Verification items for the finished model (mm, model axes). A direction names the side the tool comes from. Give positions to 0.01 mm unless a question says otherwise; leave off trailing zeros. Order: outer loops, then holes, each group sorted by start corner. A loop starts at its lowest first (then second) coordinate and runs counter-clockwise, first axis right, second up.
(1) Mould release check, pull along Y, two halves, no side actions. Record for faces 3 (the face through (-18, 24, 0)), 4 (the face through (-0.78, -22.43, -12.4)), 5 (the face through (-1, -25, -7)): pulls with the +Y half, pulls with the -Y half, needs draft (parallel to the pull), parting line crosses it, or undercut.
(2) Sectioned sample at B-B on y = -18. Record the cut outline in (x, z).
(3) Sectioned sample at A-A on z = -5. Record the cut outline in (x, y).
(4) Access from +Z, -Z, +X, -X, +Y, -Y to the whole of each face (thin tool, end or side, straight path). Record for faces 1 (the face through (-57.43, 22.4, -5.58)), 2 (the face through (60, 0, -7)).
(5) Sectioned sample at C-C on x = 18. Record the cut outline in (y, z).
(6) Scan lines: L1, parallel to X at y = -8, z = -3; L2, parallel to Y at x = -41.5, z = -7.75; L3, parallel to Z at x = 53, y = 2.5. Record each from-to range of solid material in increasing order.
(7) Gauge pin test, flat end, axial feed: pin 1 (1.5 mm diameter, centred on x = 18, y = -5.5, fed in from +Z). Record the tip position at first contact, or that the pin passes through.
```python
from build123d import *

# Parameters (mm, degrees)
SKETCH1_W           = 120
SKETCH1_H           = 50
BOSS_EXTRUDE1_DEPTH = 15
SHELL1_T            = -2
FILLET1_R           = 2


with BuildPart() as part:
    # Sketch1 → Boss-Extrude1 (new body)
    with BuildSketch(Plane.XY):
        Rectangle(SKETCH1_W, SKETCH1_H)
    extrude(amount=-BOSS_EXTRUDE1_DEPTH)

    # Shell1
    shell1_openings = [part.faces().sort_by_distance(p)[0] for p in [
        (0, 0, 0),
    ]]
    offset(amount=SHELL1_T, openings=shell1_openings, kind=Kind.INTERSECTION)

    # Fillet1
    fillet1_edges = [part.edges().sort_by_distance(p)[0] for p in [
        (58, 0, -13),
        (58, 23, -6.5),
        (0, -23, -13),
        (58, -23, -6.5),
        (-58, 0, -13),
        (-58, -23, -6.5),
        (0, 23, -13),
        (-58, 23, -6.5),
    ]]
    fillet(fillet1_edges, radius=FILLET1_R)


solid = part.part
```
Ans:
1. face 3: needs draft
1. face 4: undercut
1. face 5: pulls with the -Y half
2. outline: (-60, -15) - (60, -15) - (60, 0) - (58, 0) - (58, -11) arc R2 cw to (56, -13) - (-56, -13) arc R2 cw to (-58, -11) - (-58, 0) - (-60, 0) - close
3. outline: (-60, -25) - (60, -25) - (60, 25) - (-60, 25) - close; hole (-58, -21) arc R2 ccw to (-56, -23) - (56, -23) arc R2 ccw to (58, -21) - (58, 21) arc R2 ccw to (56, 23) - (-56, 23) arc R2 ccw to (-58, 21) - close
4. face 1: +Z
4. face 2: +Z, -Z, +X, +Y, -Y
5. outline: (-25, -15) - (25, -15) - (25, 0) - (23, 0) - (23, -11) arc R2 cw to (21, -13) - (-21, -13) arc R2 cw to (-23, -11) - (-23, 0) - (-25, 0) - close
6. L1: x = -60 to -58, 58 to 60
6. L2: y = -25 to -23, 23 to 25
6. L3: z = -15 to -13
7. pin 1: stops at z = -13
